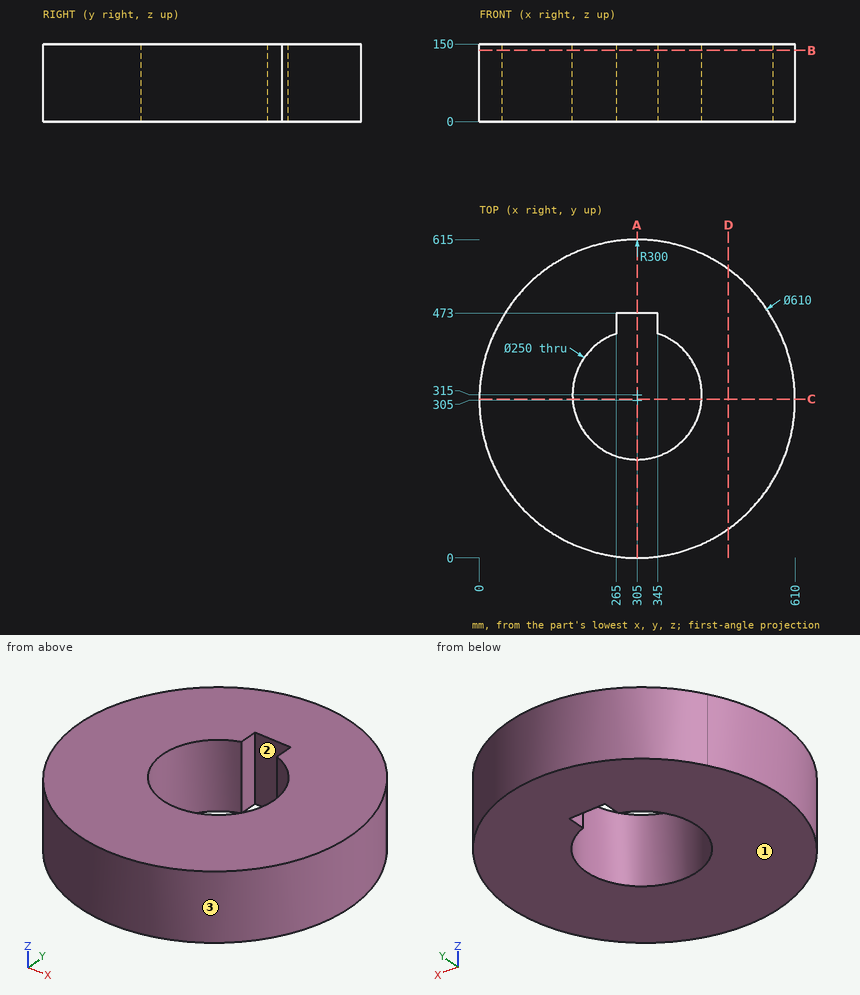
Geometry: see drawing. Coordinates: mm, zero at the bounding-box minimum. Give positions to 0.01 mm unless a question says otherwise; leave off trailing zeros. Write each loop counter-clockwise with the first axis right and the second up, starting at its lowest first coordinate (ties: lowest second). Pieces come first, ordered by that corner, then holes. Notation, with made-up numbers: (-22.75, 12) - (25.25, 12) arc R11 ccw to (25.25, 28) - close; hole circle Ø1 at (37.25, -39.75). An arc over 180 degrees is marked (long way). Return JSON: item names as keys, results as strings. Group by question number.
1) First-contact query: P1, Ø2, axis at y = 182, z = 69, coming from the -X side; P2, Ø2, axis at x = 386.5, z = 54.5, coming from the +Y side; P3, Ø12, axis at y = 461.5, z = 81.5, coming from the -X side. Flat tips, straight axial feed; report the tip coordinate or a pass-through.
2) Section C-C on y = 307. Return the cut outline in (x, z), plus the area to 3 significant figures.
3) Section D-D on x = 481.5. Return the cut outline in (y, z), plus the area to 3 significant figures.
4) Mould query, pull axis Y, two halves, no side actions, for the marked faces 1, 2 and 3. Classes: released by +Y, released by -Y, zero draft, split by the parting line, or undercut.
5) Section A-A on x = 305. Return the cut outline in (y, z), plus the area to 3 significant figures.
6) Line query: line 1 (Y direction, x = 305, z = 108); line 2 (Y direction, x = 343, z = 100.5); line 3 (X direction, y = 346, z = 92) (3 decimals). Output: solid intervals per line, ascending.
7) Section B-B on z = 137.5. Return the cut outline in (x, y).
Filled in:
{
 "1": {"P1": "stops at x = 25.46", "P2": "stops at y = 604", "P3": "stops at x = 39.72"},
 "2": {"outline": "(0.01, 0) - (180.26, 0) - (180.26, 150) - (0.01, 150) - close; (429.74, 0) - (609.99, 0) - (609.99, 150) - (429.74, 150) - close", "area": "54,100 mm^2"},
 "3": {"outline": "(56.26, 0) - (557.59, 0) - (557.59, 150) - (56.26, 150) - close", "area": "75,200 mm^2"},
 "4": {"face 1": "zero draft", "face 2": "undercut", "face 3": "split by the parting line"},
 "5": {"outline": "(0, 0) - (190, 0) - (190, 150) - (0, 150) - close; (473, 0) - (615, 0) - (615, 150) - (473, 150) - close", "area": "49,800 mm^2"},
 "6": {"line 1": "y = 0 to 190, 473 to 615", "line 2": "y = 2.38 to 195.92, 473 to 612.58", "line 3": "x = 2.768 to 183.905, 426.095 to 607.232"},
 "7": {"outline": "(43.06, 461.25) arc R305 ccw (long way) to (566.94, 461.25) arc R300 ccw to start; hole (265, 433.43) arc R125 ccw (long way) to (345, 433.43) - (345, 473) - (265, 473) - close"}
}
